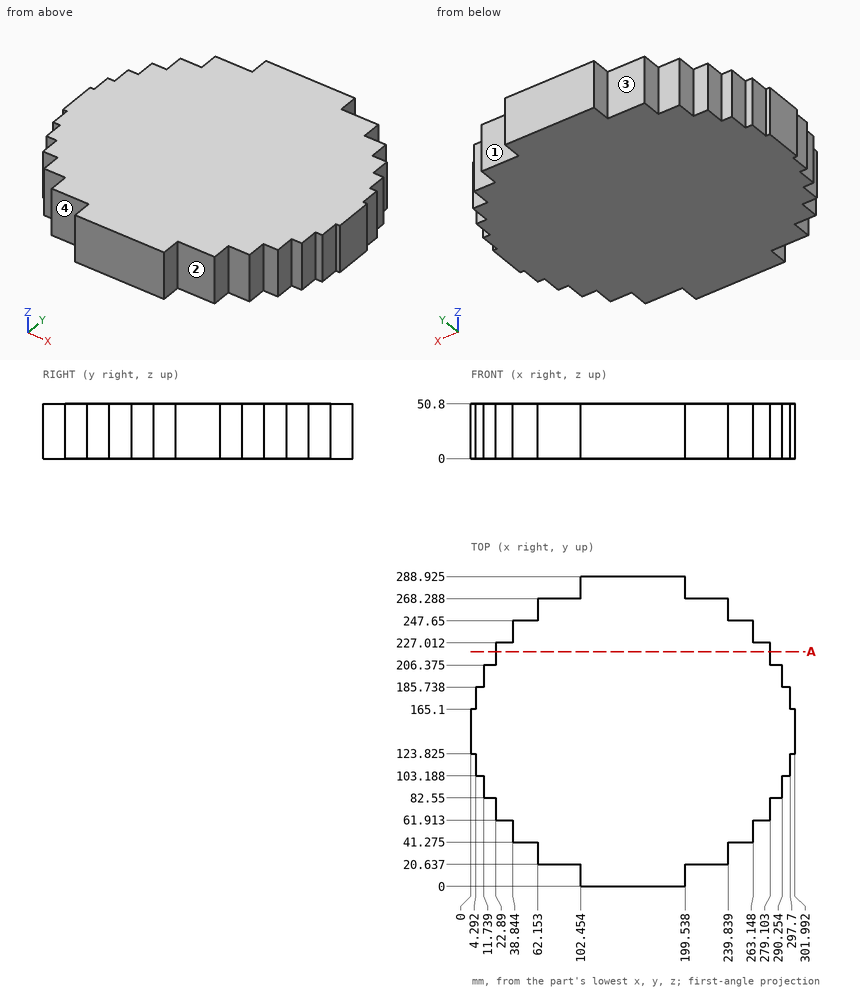
Job drawing, mm, ordinate dimensions from the low corner. One solid piece. A direction names the side the tool comes from. Coordinates: 2 decimals unless noted, no trailing zeros. Order: outer loops, then holes, each group sorted by start corner. A loop starts at its lowest first (then second) coordinate and runs counter-clockwise, first axis right, second up. Notation, with made-up numbers: (-32, -2.5) -> (20, -2.5) arc R20 ccw to (20, 14.5) -> close; hole circle Ø8 at (2.25, 70.25). An arc over 180 degrees is marked (long way). Answer in a Markdown table with one row per item. Add a question column.
Q1. Drop flat-ended pins along their axis: pin 1 (16.5 mm diameter, centred on y = 109, z = 28.5, fed in from -X); pin 2 (6 mm diameter, centred on y = 213.5, z = 23, fed in from -X); pin 3 (8 mm diameter, centred on y = 70.5, z = 32, fed in from +X). Give the stop position or say it passes through.
Q2. Band-saw the part on A-A, the plane y = 219. List the corners of the cut face in (x, z), then the cut area to 3 significant figures.
Q3. Wall check: line 1 along X through (y, z) = (102.5, 21.5); line 2 along X through (y, z) = (261.5, 31); line 3 along Y through (x, z) = (85, 32). Give the ranges that are in metal, low to high. Write a range as [from, to].
Q4. Which spindle directions (+Z, -Z, +X, -X, +Y, -Y) get a long thin tool onto all of the face, cutting with end or side? Do the marked faces 1, 2, 3 and 4. Say none if no direction does.
Answers follow:
| question | item | result |
|---|---|---|
| 1 | pin 1 | x = 4.29 |
| 1 | pin 2 | x = 22.89 |
| 1 | pin 3 | x = 279.1 |
| 2 | outline | (22.89, 0) -> (279.1, 0) -> (279.1, 50.8) -> (22.89, 50.8) -> close |
| 2 | area | 13,000 mm^2 |
| 3 | line 1 | [11.74, 290.25] |
| 3 | line 2 | [62.15, 239.84] |
| 3 | line 3 | [20.64, 268.29] |
| 4 | face 1 | +Z, -Z, +X, +Y |
| 4 | face 2 | +Z, -Z, +X, -Y |
| 4 | face 3 | +Z, -Z, -X, +Y |
| 4 | face 4 | +Z, -Z, -X, -Y |
